Design review of the part built by this model. Coordinates are the model's own, in mm. A direction names the side the tool comes from. Coordinates: 2 decimals unless noted, no trailing zeros. Loops run counter-clockwise (first coordinate to the right, second up) from the corner with the lowest first, then second, coordinate; pieces in that order, holes last.
Q1. Machinability: for faces 1 (the face through (0, 0, 0)), 2 (the face through (-1.625, 16, 8)), 3 (the face through (0, 16, 7.375)), 4 (the face through (-6.324, 5.437, -4.032)), 5 (the face through (-6.324, 42.846, -4.032)), which of the approach directions +Z, -Z, +X, -X, +Y, -Y give a long, thin tool a straight path to every point of the face, cutting with its end or side? Answer none if there is none.
Q2. Add section D-D on y = 29.5. Give the boundary of the cut face in (x, z).
Q3. Draft analysis for pull direction X (two halves, no side actions). For faces 6 (the face through (1.625, 16, 8)), 7 (the face through (-5, 10, -6)), 8 (the face through (-12.65, 26.94, -8.06)), state which applies: released by +X, released by -X, zero draft, split by the parting line, or undercut.
Q4. Add section A-A on z = 0. Give the boundary of the cut face in (x, y).
Q5. Add section C-C on y = 13. Give the boundary of the cut face in (x, z) (3 decimals).
Q6. For P1, Ø14, axis at x = 0.5, z = -7, coming from the +Y side; P2, Ø2.5, axis at x = 0, y = 17.5, coming from the +Z side (3 decimals); P3, Ø1, axis at x = -3, z = -10, coming from the -Y side; P4, Ø1.5, axis at x = 1, y = 17.5, coming from the +Z side, all flat-tipped, find the tip position at first contact; note any pin that passes through.
Q7. Wall thickness on probe 1 along Y at (x, z) = (-5.5, -12.25); probe 2 along X at (y, z) = (12.5, 7.75) (3 decimals); probe 3 along X at (y, z) = (24, 12): over which ranges is each line inside the solid? List them lowest first.
Q8. Add section B-B on x = 0. Give the boundary of the cut face in (y, z) (3 decimals).
```python
from build123d import *

# Parameters (mm, degrees)
SKETCH2_W          = 3.25
SKETCH2_H          = 3.25
CUT_EXTRUDE1_DEPTH = 12
CHAMFER1_SIZE      = 1


with BuildPart() as part:
    # Sketch1 → Revolve1 (revolve)
    with BuildSketch(Plane.XY, mode=Mode.PRIVATE) as revolve1_sk:
        Polygon((0, 0), (0, 55), (7.5, 55), (7.5, 32), (15, 32), (15, 22), (9, 22), (9, 10), (7.5, 10), (7.5, 0), align=None)
    revolve(revolve1_sk.sketch.rotate(Axis((0, 0, 0), (0, 1, 0)), 90), axis=Axis((0, 0, 0), (0, 1, 0)))

    # Sketch2 → Cut-Extrude1 (cut)
    with BuildSketch(Plane.XZ.offset(-10)):
        with Locations((0, 9)):
            Rectangle(SKETCH2_W, SKETCH2_H)
    extrude(amount=-CUT_EXTRUDE1_DEPTH, mode=Mode.SUBTRACT)

    # Chamfer1
    chamfer1_edges = [part.edges().sort_by_distance(p)[0] for p in [
        (0, 55, 7.5),
        (0, 10, -9),
        (0, 0, 7.5),
        (0, 22, 15),
        (0, 32, 15),
    ]]
    chamfer(chamfer1_edges, length=CHAMFER1_SIZE)


solid = part.part
```
Entries:
1. face 1: +Z, -Z, +X, -X, -Y
1. face 2: +Z, -Y
1. face 3: +Z
1. face 4: -Y
1. face 5: +Y
2. outline: circle Ø30 at (0, 0)
3. face 6: undercut
3. face 7: zero draft
3. face 8: split by the parting line
4. outline: (-15, 23) - (-14, 22) - (-9, 22) - (-9, 11) - (-8, 10) - (-7.5, 10) - (-7.5, 1) - (-6.5, 0) - (6.5, 0) - (7.5, 1) - (7.5, 10) - (8, 10) - (9, 11) - (9, 22) - (14, 22) - (15, 23) - (15, 31) - (14, 32) - (7.5, 32) - (7.5, 54) - (6.5, 55) - (-6.5, 55) - (-7.5, 54) - (-7.5, 32) - (-14, 32) - (-15, 31) - close
5. outline: (-1.625, 7.375) - (-1.625, 8.852) arc R9 ccw (long way) to (1.625, 8.852) - (1.625, 7.375) - close
6. P1: stops at y = 55
6. P2: stops at z = 7.375
6. P3: stops at y = 22
6. P4: stops at z = 8.85
7. probe 1: y = 22 to 32
7. probe 2: x = -4.576 to -1.625, 1.625 to 4.576
7. probe 3: x = -9 to 9
8. outline: (0, -6.5) - (1, -7.5) - (10, -7.5) - (10, -8) - (11, -9) - (22, -9) - (22, -14) - (23, -15) - (31, -15) - (32, -14) - (32, -7.5) - (54, -7.5) - (55, -6.5) - (55, 6.5) - (54, 7.5) - (32, 7.5) - (32, 14) - (31, 15) - (23, 15) - (22, 14) - (22, 7.375) - (10, 7.375) - (10, 7.5) - (1, 7.5) - (0, 6.5) - close
